Read the model definition and answer for the solid it produces. Units are mm, in the model's axes. Face numbers are marked on the shaded views. A direction names the side the tool comes from. Coordinates: 2 decimals unless noted, no trailing zeros. Write each loop counter-clockwise with the first axis right and the second up, starting at its lowest first coordinate (ties: lowest second). Pieces come first, ordered by that corner, then holes.
1) Which of the six approach directions +Z, -Z, +X, -X, +Y, -Y give full straight-line access (tool end or side, diameter ignored) to the marked faces 1 and 2?
2) Find the intervals of material crossed by line 1 (X direction, y = 24, z = 17.5) (3 decimals); line 2 (Y direction, x = 24.25, z = 12.7), in increasing order.
3) Determine the mould class of the marked faces 3, 4, 5 and 6 for opening direction X: +X half, -X half, draft (parallel to the pull), parting line (faces both ways), or undercut.
4) The part is cut by section B-B (x = 5). Determine the outline of the cut face in (y, z) (3 decimals).
5) The part is cut by section C-C (z = 75.5). Determine the outline of the cut face in (x, y) (3 decimals).
6) The part is cut by section A-A (y = 12.7). Determine the outline of the cut face in (x, z) (1 decimal), then the cut area to 3 significant figures.
7) Each of these flat-tipped pins is pushed along its axis until it touches: pin 1 Ø1.6 at (x, y) = (17, 23.5) entering from -Z; pin 2 Ø7.5 at (y, z) = (12.7, 12.7) entering from -X. Where does it stop, or does it pass through?
8) The part is cut by section D-D (y = 4). Determine the outline of the cut face in (x, z) (3 decimals).
Autodesk Inventor part; units mm, degrees
ref_plane "YZ Plane" through (0, 0, 0) normal (1, 0, 0) x (0, 1, 0)
ref_plane "XZ Plane" through (0, 0, 0) normal (0, 1, 0) x (-1, 0, 0)
ref_plane "XY Plane" through (0, 0, 0) normal (0, 0, 1) x (1, 0, 0)
sketch "Sketch1" plane through (0, 0, 0) normal (0, 0, 1) x (1, 0, 0)
  line L0 (0, 0) -> (25.4, 0)
  line L1 (25.4, 0) -> (25.4, 25.4)
  line L2 (25.4, 25.4) -> (0, 25.4)
  line L3 (0, 25.4) -> (0, 0)
  line L4 (3.175, 3.175) -> (22.225, 3.175)
  line L5 (22.225, 3.175) -> (22.225, 22.225)
  line L6 (22.225, 22.225) -> (3.175, 22.225)
  line L7 (3.175, 22.225) -> (3.175, 3.175)
  dimension "d0" = 25.4
  dimension "d1" = 25.4
  dimension "d2" = 3.175
  dimension "d3" = 3.175
  dimension "d4" = 3.175
  dimension "d5" = 3.175
extrude "Extrusion1" add sketch "Sketch1" along normal blind 85.725
sketch "Sketch2" plane through (25.4, 0, 0) normal (1, 0, 0) x (0, 0, -1)
  line L0 (-85.725, 25.4) -> (-85.725, 0)
  line L1 (0, 0) -> (-85.725, 0)
  line L2 (0, 0) -> (0, 25.4)
  line L3 (0, 25.4) -> (-85.725, 25.4)
  circle A0 centre (-12.7, 12.7) radius 4.7625
  arc A1 (-12.7, 0) -> (-12.7, 25.4) centre (-12.7, 12.7) ccw
  dimension "d8" = 9.525
  dimension "d9" = 12.7
  dimension "d10" = 12.7
extrude "Extrusion2" cut sketch "Sketch2" against normal blind 25.4 contours L3 L2 A1 | A1 L2 L1 | A0
sketch "Sketch3" plane through (0, 25.4, 85.725) normal (0, 1, 0) x (1, 0, 0)
  line L0 (0, 73.025) -> (25.4, 73.025)
  line L1 (3.175, 82.55) -> (22.225, 82.55)
  line L2 (22.225, 82.55) -> (22.225, 66.675)
  line L3 (22.225, 66.675) -> (3.175, 66.675)
  line L4 (3.175, 66.675) -> (3.175, 82.55)
  line L5 (0, 85.725) -> (0, 73.025)
  dimension "d13" = 19.05
  dimension "d14" = 3.175
  dimension "d17" = 15.875
  dimension "d18" = 6.35
extrude "Extrusion3" cut sketch "Sketch3" against normal through all
equation "\"d2\" = d5"
equation "\"d3\" = d2"
equation "\"d5\" = d4"
equation "\"d10\" = d9"
properties part number "8 ball pnumatic arm tube"
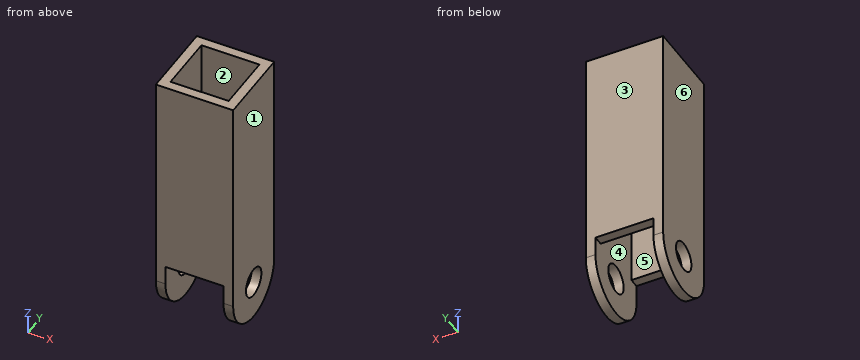
Reported:
1. face 1: +Z, -Z, +X, +Y, -Y
1. face 2: +Z, -Z
2. line 1: x = 0 to 3.175, 22.225 to 25.4
2. line 2: y = 0 to 7.94, 17.46 to 25.4
3. face 3: draft
3. face 4: undercut
3. face 5: undercut
3. face 6: -X half
4. outline: (0, 19.05) - (3.175, 19.05) - (3.175, 85.725) - (0, 85.725) - close; (22.225, 19.05) - (25.4, 19.05) - (25.4, 85.725) - (22.225, 85.725) - close
5. outline: (0, 0) - (25.4, 0) - (25.4, 25.4) - (0, 25.4) - close; hole (3.175, 3.175) - (22.225, 3.175) - (22.225, 22.225) - (3.175, 22.225) - close
6. outline: (0, 0) - (3.2, 0) - (3.2, 7.9) - (0, 7.9) - close; (0, 17.5) - (3.2, 17.5) - (3.2, 85.7) - (0, 85.7) - close; (22.2, 0) - (25.4, 0) - (25.4, 7.9) - (22.2, 7.9) - close; (22.2, 17.5) - (25.4, 17.5) - (25.4, 85.7) - (22.2, 85.7) - close
6. area: 484 mm2
7. pin 1: stops at z = 19.05
7. pin 2: passes through
8. outline: (0, 3.448) - (3.175, 3.448) - (3.175, 85.725) - (0, 85.725) - close; (22.225, 3.448) - (25.4, 3.448) - (25.4, 85.725) - (22.225, 85.725) - close
